Autodesk Inventor part; units mm, degrees
ref_plane "YZ Plane" through (0, 0, 0) normal (1, 0, 0) x (0, 1, 0)
ref_plane "XZ Plane" through (0, 0, 0) normal (0, 1, 0) x (-1, 0, 0)
ref_plane "XY Plane" through (0, 0, 0) normal (0, 0, 1) x (1, 0, 0)
sketch "Sketch1" plane through (0, 0, 0) normal (0, 0, 1) x (1, 0, 0)
  line L0 (0, 0) -> (0, -19.05) construction
  line L1 (0, -19.05) -> (19.05, -19.05) construction
  circle A0 centre (0, 0) radius 2.3813
  circle A1 centre (19.05, -19.05) radius 3.9687
  circle A2 centre (0, 0) radius 4.7625
  circle A3 centre (19.05, -19.05) radius 12.7
  line L2 (0, 0) -> (19.05, -19.05) construction
  line L3 (-4.3763, -1.912) -> (11.0982, -31.1817)
  line L4 (1.2997, 4.7) -> (30.5694, -10.7745)
  point P0 (7.7583, -1.6771)
  point P1 (-4.2103, -2.2259)
  point P2 (7.8225, -24.9858)
  point P3 (24.9858, -7.8225)
  point P4 (2.2259, 4.2103)
  dimension "d0" = 19.05
  dimension "d1" = 19.05
  dimension "d2" = 4.7625
  dimension "d3" = 7.9375
  dimension "d4" = 9.525
  dimension "d5" = 25.4
extrude "Extrusion1" add sketch "Sketch1" along normal blind 1.5875
properties part number "pto"
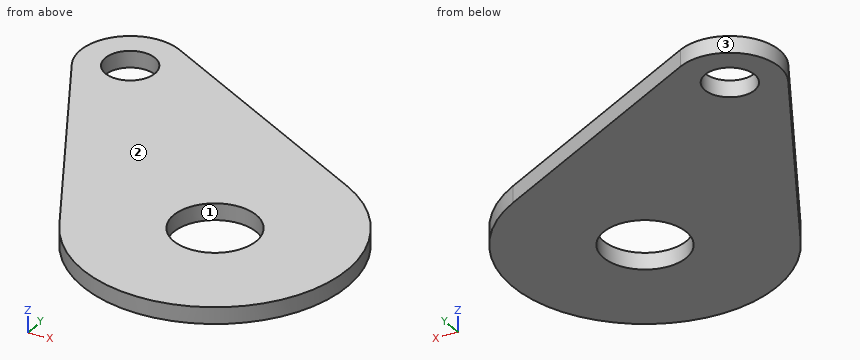
Build history of the part. All positions in model axes, mm. Face numbers are marked on the shaded views. Give positions to 0.01 mm unless a question says otherwise; leave off trailing zeros. Order: outer loops, then holes, each group sorted by start corner. A loop starts at its lowest first (then second) coordinate and runs counter-clockwise, first axis right, second up. Notation, with made-up numbers: M 83,38 L 111,38 A23 ccw 111,60 Z; hole C 35.25,45 d2. An arc over 180 degrees is marked long. Use one line per item in the form item = value.
Q1. Slice it at B-B, the plane x = 0. Write the cut outline in (y, z).
Conclusion:
outline = M -10.19,0 L -2.38,0 L -2.38,1.59 L -10.19,1.59 Z; M 2.38,0 L 4.76,0 L 4.76,1.59 L 2.38,1.59 Z
Q2. Pull direction X, two halves, no side cores. Call the marked faces 1, 2 and 3: released by +X, released by -X, zero draft, split by the parting line, or undercut.
Conclusion:
face_1 = undercut
face_2 = zero draft
face_3 = split by the parting line
Q3. Slice it at C-C, the plane z = 0.35. State how many separate pieces and enclosed holes the cut face has, and give its area (3 significant figures).
Conclusion:
separate_pieces = 1
enclosed_holes = 2
area = 713 mm2
Q4. Wall check: probe 1 along Y at (x, z) = (0, 0.65); probe 2 along Y at (x, z) = (-0.5, 0.7); probe 3 along X at (y, z) = (1, 0.6). Give the ranges that are in metal, low to high.
Conclusion:
probe_1 = -10.19 to -2.38, 2.38 to 4.76
probe_2 = -9.24 to -2.33, 2.33 to 4.74
probe_3 = -4.66 to -2.16, 2.16 to 8.3
Q5. Slice it at D-D, the plane y = -26.5. Write the cut outline in (x, z), and give its area (3 significant figures).
Conclusion:
outline = M 8.76,0 L 29.34,0 L 29.34,1.59 L 8.76,1.59 Z
area = 32.7 mm2
Q6. Slice it at A-A, the plane y = -21. Write the cut outline in (x, z), and give its area (3 significant figures).
Conclusion:
outline = M 5.72,0 L 15.59,0 L 15.59,1.59 L 5.72,1.59 Z; M 22.51,0 L 31.6,0 L 31.6,1.59 L 22.51,1.59 Z
area = 30.1 mm2
